For this review, use the dimensioned drawing (mm, ordinates from the lowest corner) and the shaded views. Coordinates: 2 decimals unless noted, no trailing zeros. Write each loop counter-clockwise with the first axis right and the second up, starting at its lowest first coordinate (ties: lowest second). Pieces come first, ordered by that corner, then holes. Notation, with made-up numbers: (6.25, -12) - (15.25, -12) arc R29 ccw to (15.25, 8) - close; hole circle Ø8 at (22.5, -24.5). An arc over 180 degrees is marked (long way). Use one line per item in the form item = value. Start each with the question number.
1) We need section D-D (y = 15). Give the boundary of the cut face in (x, z), plus the area to 3 significant figures.
2) For L1, parallel to Z at x = 63.5, y = 18.25; L2, parallel to Z at x = 38.1, y = 9; L3, parallel to X at y = 10.75, z = 41.5 (1 decimal), list the stretches that pass through material, from the lowest coordinate up. Write a range as from..to.
3) We need section A-A (x = 38.1). Give the boundary of the cut face in (y, z).
4) Mouldability with a two-part tool opening along Z and no side actions: class the marked faces 1, 2 and 3 as pulls with the +Z half, pulls with the -Z half, needs draft (parallel to the pull), parting line crosses it, or undercut.
5) We need section B-B (x = 12.7). Give the boundary of the cut face in (y, z), plus the area to 3 significant figures.
6) We need section C-C (z = 40). Give the boundary of the cut face in (x, y).
7) Insertion check: P1, Ø1.5, axis at x = 57, z = 64.5, coming from the -Y side. The pin has a flat end and moves straight along its axis. Give the tip position at first contact, or say it passes through.
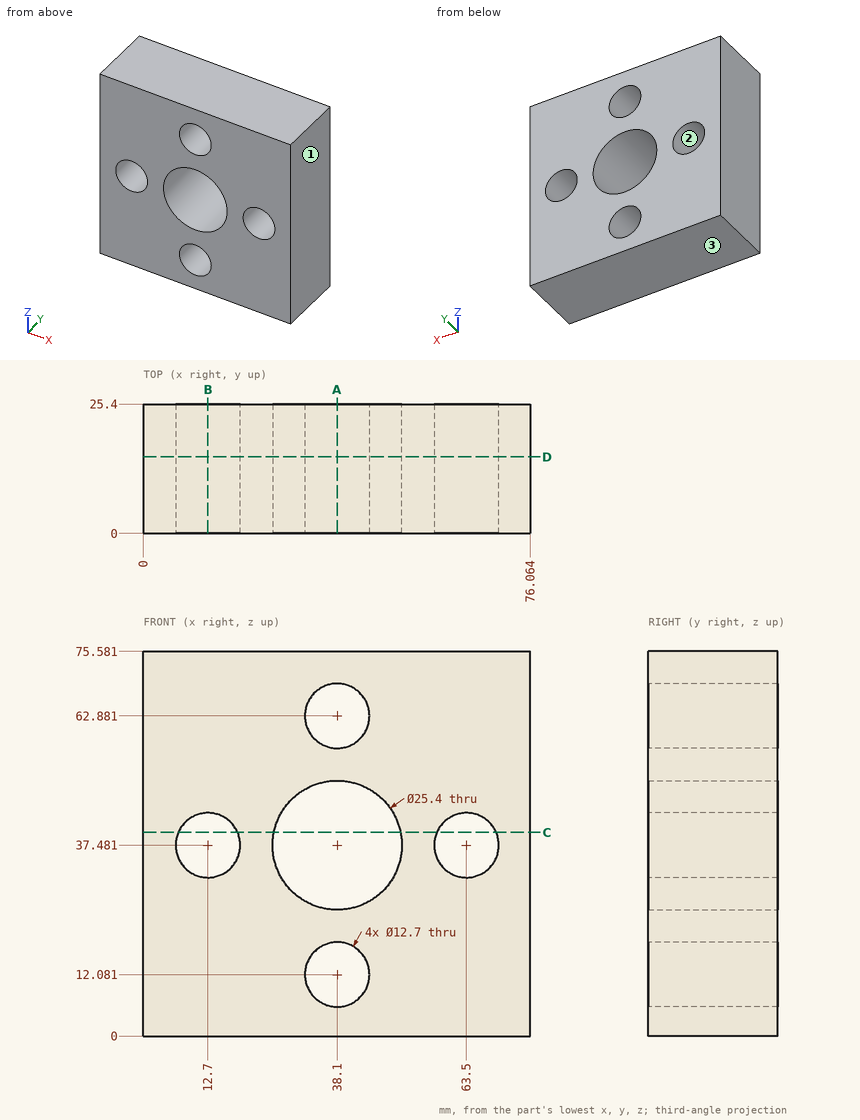
Determined:
q1.outline = (0, 0) - (76.06, 0) - (76.06, 75.58) - (0, 75.58) - close; hole circle Ø12.7 at (12.7, 37.48); hole circle Ø25.4 at (38.1, 37.48); hole circle Ø12.7 at (38.1, 12.08); hole circle Ø12.7 at (38.1, 62.88); hole circle Ø12.7 at (63.5, 37.48)
q1.area = 4,740 mm²
q2.L1 = 0..31.13, 43.83..75.58
q2.L2 = 0..5.73, 18.43..24.78, 50.18..56.53, 69.23..75.58
q2.L3 = 0..7.8, 17.6..26.1, 50.1..58.6, 68.4..76.1
q3.outline = (0, 0) - (25.4, 0) - (25.4, 5.73) - (0, 5.73) - close; (0, 18.43) - (25.4, 18.43) - (25.4, 24.78) - (0, 24.78) - close; (0, 50.18) - (25.4, 50.18) - (25.4, 56.53) - (0, 56.53) - close; (0, 69.23) - (25.4, 69.23) - (25.4, 75.58) - (0, 75.58) - close
q4.face_1 = needs draft
q4.face_2 = undercut
q4.face_3 = pulls with the -Z half
q5.outline = (0, 0) - (25.4, 0) - (25.4, 31.13) - (0, 31.13) - close; (0, 43.83) - (25.4, 43.83) - (25.4, 75.58) - (0, 75.58) - close
q5.area = 1,600 mm²
q6.outline = (0, 0) - (6.87, 0) - (6.87, 25.4) - (0, 25.4) - close; (18.53, 0) - (25.65, 0) - (25.65, 25.4) - (18.53, 25.4) - close; (50.55, 0) - (57.67, 0) - (57.67, 25.4) - (50.55, 25.4) - close; (69.33, 0) - (76.06, 0) - (76.06, 25.4) - (69.33, 25.4) - close
q7.P1 = 0
